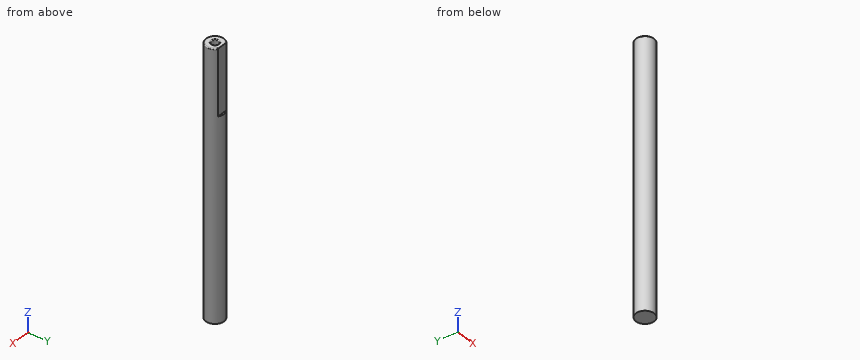
from build123d import *

# Parameters (mm, degrees)
SKETCH1_R          = 2.5
EXTRUDE1_DEPTH     = 73
SKETCH2_R          = 1
ICE1_DEPTH         = 10
FILLET1_R          = 0.25
CUT_EXTRUDE1_DEPTH = 18


with BuildPart() as part:
    # Sketch1 → Extrude1 (new body)
    with BuildSketch(Plane.XY):
        Circle(SKETCH1_R)
    extrude(amount=EXTRUDE1_DEPTH)

    # Sketch2 → ICE1 (cut)
    with BuildSketch(Plane.XY.offset(73)):
        Circle(SKETCH2_R)
    extrude(amount=-ICE1_DEPTH, mode=Mode.SUBTRACT)

    # Fillet1
    fillet1_edges = [part.edges().sort_by_distance(p)[0] for p in [
        (-2.5, 0, 73),
        (-1, 0, 73),
    ]]
    fillet(fillet1_edges, radius=FILLET1_R)

    # Sketch4 → Cut-Extrude1 (cut)
    with BuildSketch(Plane.XY.offset(73)):
        with BuildLine():
            Line((-1.5, 2), (1.5, 2))
            ThreePointArc((1.5, 2), (0, 2.5), (-1.5, 2))
        make_face()
    extrude(amount=-CUT_EXTRUDE1_DEPTH, mode=Mode.SUBTRACT)


solid = part.part
Geometry: final body of the model. Coordinates: model frame, mm. Round coordinates to 2 decimals unless told otherwise and drop trailing zeros. Loops run counter-clockwise (first coordinate to the right, second up) from the corner with the lowest first, then second, coordinate; pieces in that order, holes last. Notation, with made-up numbers: M 19,22.25 L 60,22.25 A30 ccw 60,57.25 Z; hole C 18.5,44 d10. An arc over 180 degrees is marked long. Put each result on its own line as item: value. Start each with the question number.
(1) Section query C-C (z = 45.5). Return loops of the section in (x, y), then the cut area to 3 significant figures.
(2) Section query A-A (y = 0). Return loops of the section in (x, z).
(3) Material intervals for line 1 along Z through (x, y) = (0.95, 2.2); line 2 along Z through (x, y) = (-0.3, -0.6); line 3 along X through (y, z) = (0.2, 46.5), sorted ascending. Write a range as [from, to].
(4) Section query B-B (x = 0). Return loops of the section in (y, z).
(5) Contact query for flat-ended pins moving along their axis: pin 1 Ø1.5 at (x, z) = (-1.5, 21.5) entering from -Y; pin 2 Ø1 at (y, z) = (-2, 9.5) entering from +X; pin 3 Ø1.5 at (x, z) = (1, 31) entering from -Y. Output: stop coordinate, or through.
Findings below:
1. outline: C 0,0 d5
1. area: 19.6 mm2
2. outline: M -2.5,0 L 2.5,0 L 2.5,72.75 A0.25 ccw 2.25,73 L 1.25,73 A0.25 ccw 1,72.75 L 1,63 L -1,63 L -1,72.75 A0.25 ccw -1.25,73 L -2.25,73 A0.25 ccw -2.5,72.75 Z
3. line 1: z = [0, 55]
3. line 2: z = [0, 63]
3. line 3: x = [-2.49, 2.49]
4. outline: M -2.5,0 L 2.5,0 L 2.5,55 L 2,55 L 2,73 L 1.25,73 A0.25 ccw 1,72.75 L 1,63 L -1,63 L -1,72.75 A0.25 ccw -1.25,73 L -2.25,73 A0.25 ccw -2.5,72.75 Z
5. pin 1: stops at y = -2.38
5. pin 2: stops at x = 2
5. pin 3: stops at y = -2.49
